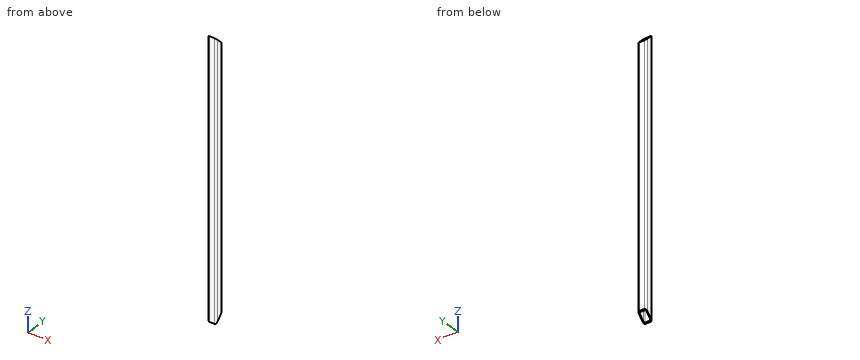
Autodesk Inventor part; units mm, degrees
ref_plane "Start Plane" through (0, 0, -15) normal (0, 0, 1) x (1, 0, 0)
ref_plane "End Plane" through (0, 0, 987) normal (0, 0, 1) x (1, 0, 0)
ref_plane "Work Plane6" through (0, -15, 987) normal (0, 0.7071, 0.7071) x (1, 0, 0)
ref_plane "Start Plane" through (0, 0, -15) normal (0, 0, 1) x (1, 0, 0)
ref_plane "End Plane" through (0, 0, 987) normal (0, 0, 1) x (1, 0, 0)
sketch "Sketch" plane through (0, 0, 0) normal (0, 0, 1) x (1, 0, 0)
  line L0 (-15, -9) -> (-15, 9)
  line L1 (-9, 15) -> (9, 15)
  line L2 (15, 9) -> (15, -9)
  line L3 (9, -15) -> (-9, -15)
  arc A0 (-15, -9) -> (-9, -15) centre (-9, -9) ccw
  arc A1 (-9, 15) -> (-15, 9) centre (-9, 9) ccw
  arc A2 (15, 9) -> (9, 15) centre (9, 9) ccw
  arc A3 (9, -15) -> (15, -9) centre (9, -9) ccw
  arc A4 (-9, 12) -> (-12, 9) centre (-9, 9) ccw
  line L4 (-9, 12) -> (9, 12)
  arc A5 (12, 9) -> (9, 12) centre (9, 9) ccw
  line L5 (12, 9) -> (12, -9)
  arc A6 (9, -12) -> (12, -9) centre (9, -9) ccw
  line L6 (9, -12) -> (-9, -12)
  arc A7 (-12, -9) -> (-9, -12) centre (-9, -9) ccw
  line L7 (-12, -9) -> (-12, 9)
  line L8 (0, 22.7397) -> (0, -22.7397) construction
  line L9 (-22.7397, 0) -> (22.7397, 0) construction
  dimension "d7" = 6
  dimension "d10" = 30
  dimension "d11" = 30
  dimension "d12" = 3
  dimension "d15" = 15
  dimension "d16" = 15
extrude "Body" add sketch "Sketch" along normal up to surface (1002 mm away) from surface at -15
sketch "Sketch3" plane through (0, 0, 0) normal (0, 0, 1) x (1, 0, 0)
  line L0 (0, 0) -> (10, 0)
ref_plane "Work Plane3" through (0, 0, 0) normal (0, -1, 0) x (1, 0, 0)
ref_plane "Work Plane6" through (0, -15, 987) normal (0, 0.7071, 0.7071) x (1, 0, 0)
split "Split3" plane through (0, -15, 987) removes the side toward (0, 0.7071, 0.7071)
ref_plane "Work Plane7" through (-0.0002, -15, -15) normal (0, 0.7071, -0.7071) x (1, 0, 0)
split "Split4" plane through (-0.0002, -15, -15) removes the side toward (0, 0.7071, -0.7071)
sketch "Sketch4" plane through (0, 0, 0) normal (0, -1, 0) x (1, 0, 0)
  line L0 (-2, -15) -> (12, -15)
  line L1 (-2, 987) -> (12, 987)
  dimension "d18" = 1002
equation "\"d7\" = G_IR"
equation "\"d10\" = G_H"
equation "\"d11\" = G_W"
equation "\"d12\" = G_T"
equation "\"d15\" = 0.5 * d10"
equation "\"d16\" = 0.5 * d11"
equation "\"d3\" = G_L"
equation "\"G_W\" = 30"
equation "\"G_H\" = 30"
equation "\"G_T\" = 3"
equation "\"G_IR\" = 6"
equation "\"G_L\" = d18"
equation "\"G_OFFSET_START\" = 14.99997"
equation "\"G_OFFSET_END\" = 15"
equation "\"d13\" = -G_OFFSET_START"
equation "\"d14\" = G_OFFSET_END + B_L"
equation "\"B_L\" = 972"
properties part number "DIN EN 10219-2 - 30 x 30 x 3  - 1002" material "Steel, Mild"
The listing builds one solid part. Answer for the finished solid, in the listing's coordinates (mm). Coordinates: 2 decimals unless noted, no trailing zeros. Loops run counter-clockwise (first coordinate to the right, second up) from the corner with the lowest first, then second, coordinate; pieces in that order, holes last. Notation, with made-up numbers: M 37.25,54 L 63.25,54 A27 cw 63.25,93 Z; hole C -7,20 d8. An arc over 180 degrees is marked long. Answer as a JSON object with one key per item and string values. Group by question number.
Item 1: Section A-A (x = 0.75) is taken. Write down the section's boundary in (y, z), and give its area (3 significant figures).
Item 2: Section B-B (y = -3) is taken. Write down the section's boundary in (x, z).
Item 3: Consider L1, parallel to X at y = -7.5, z = 647.5; L2, parallel to Y at x = 10, z = 481. Determine where each line is inside the solid, lowest interval first.
Item 4: Section C-C (z = 364.5) is taken. Write down the section's boundary in (x, y), and give its area (3 significant figures).
Item 5: Each of these flat-tipped pins is pushed along its axis until it touches: P1, Ø8, axis at x = 11, y = -3, coming from the +Z side; P2, Ø1, axis at y = -10.5, z = 510, coming from the +X side; P3, Ø2, axis at x = 11, z = 619.5, coming from the +Y side. Where does it stop, or does it pass through?
Solved:
{
 "1": {"outline": "M -15,-15 L -12,-12 L -12,984 L -15,987 Z; M 12,12 L 15,15 L 15,957 L 12,960 Z", "area": "5,830 mm2"},
 "2": {"outline": "M -15,-3 L -12,-3 L -12,975 L -15,975 Z; M 12,-3 L 15,-3 L 15,975 L 12,975 Z"},
 "3": {"L1": "x = -15 to -12, 12 to 15", "L2": "y = -14.92 to -11.83, 11.83 to 14.92"},
 "4": {"outline": "M -15,-9 A6 ccw -9,-15 L 9,-15 A6 ccw 15,-9 L 15,9 A6 ccw 9,15 L -9,15 A6 ccw -15,9 Z; hole M -12,-9 A3 ccw -9,-12 L 9,-12 A3 ccw 12,-9 L 12,9 A3 ccw 9,12 L -9,12 A3 ccw -12,9 Z", "area": "301 mm2"},
 "5": {"P1": "stops at z = 978.87", "P2": "stops at x = 14.92", "P3": "stops at y = 14.92"}
}
